```python
from build123d import *

# Parameters (mm, degrees)
SKETCH1_R           = 19.05
BOSS_EXTRUDE1_DEPTH = 12.7
SKETCH2_W           = 12.7
SKETCH2_H           = 2.54
SKETCH3_R           = 2.667
CUT_EXTRUDE1_DEPTH  = 30.784140075
BOSS_EXTRUDE2_DEPTH = 2.54
BOSS_EXTRUDE2_TAPER = 20
CIRPATTERN1_COUNT   = 6


with BuildPart() as part:
    # Sketch1 → Boss-Extrude1 (new body)
    with BuildSketch(Plane.XY):
        Circle(SKETCH1_R)
    extrude(amount=BOSS_EXTRUDE1_DEPTH)

    # Sketch2 → Cut-Revolve1 (revolve, cut)
    with BuildSketch(Plane(origin=(0, 0, 0), x_dir=(1, 0, 0), z_dir=(0, 1, 0)), mode=Mode.PRIVATE) as cut_revolve1_sk:
        with Locations((12.7, -6.35)):
            Rectangle(SKETCH2_W, SKETCH2_H)
    revolve(cut_revolve1_sk.sketch.rotate(Axis((0, 0, 0), (0, 0, 1)), 180), axis=Axis((0, 0, 0), (0, 0, 1)), mode=Mode.SUBTRACT)

    # Sketch3 → Cut-Extrude1 (cut, through all)
    with BuildSketch(Plane.XY.offset(12.7)):
        Circle(SKETCH3_R)
    extrude(amount=-CUT_EXTRUDE1_DEPTH, mode=Mode.SUBTRACT)

    # Sketch4 → Boss-Extrude2 (add)
    with BuildSketch(Plane(origin=(0, 0, 0), x_dir=(-1, 0, 0), z_dir=(0, 0, -1))):
        Polygon((-4.445, 3.050443212), (-2.54, 6.35), (-4.445, 9.649556788), (-8.255, 9.649556788), (-10.16, 6.35), (-8.255, 3.050443212), align=None)
    boss_extrude2 = extrude(amount=BOSS_EXTRUDE2_DEPTH, taper=BOSS_EXTRUDE2_TAPER)

    # CirPattern1: Boss-Extrude2 ×6 about axis
    cirpattern1_axis = Axis((0, 0, 0), (0, 0, 1))
    for i in range(1, CIRPATTERN1_COUNT):
        add(boss_extrude2.rotate(cirpattern1_axis, i * 360 / CIRPATTERN1_COUNT))


solid = part.part
```
Geometry: final body of the model. Coordinates: model frame, mm. A direction names the side the tool comes from. Give positions to 0.01 mm unless a question says otherwise; leave off trailing zeros. Order: outer loops, then holes, each group sorted by start corner. A loop starts at its lowest first (then second) coordinate and runs counter-clockwise, first axis right, second up. Notation, with made-up numbers: M 43.5,9.5 L 48.5,9.5 A18 ccw 48.5,31.5 Z; hole C -3.5,52 d8. An arc over 180 degrees is marked long. Answer as CSV lines item,"result". Start each with the question number.
1) Cut plane B-B (z = 1). Output: boundary loops of the cut face in (x, y), then the cut area to 3 significant figures.
2) First-contact query: P1, Ø4, axis at x = 8.5, z = 3.5, coming from the -Y side; P2, Ø6, axis at y = 6.5, z = 5, coming from the -X side; P3, Ø4, axis at x = 14, y = -11, coming from the -Z side. Flat tips, straight axial feed; report the tip coordinate or a pass-through.
3) Cut plane A-A (z = 6.25). Output: boundary loops of the cut face in (x, y).
4) Line query: line 1 (Z direction, x = 1.5, y = 7); line 2 (Y direction, x = 0, z = 5.25); line 3 (Y direction, x = 0, z = 8.5). Output: solid intervals per line, ascending. Write a range as from..to.
5) Set-up query: faces 1 (the flat face through (4, 0, 0)), 2 (the flat face through (-2, 9, -2.54)), 3 (the cylindrical face through (-2.93, 5.634, 6.332)). Return all of +Z, -Z, +X, -X, +Y, -Y with unobstructed straight access to the full face (end or side cutting, diameter ignored); none if empty.
6) Mould query, pull axis Z, two halves, no side actions, for faces 4 (the cylindrical face through (-15.12, -11.59, 2.5)), 5 (the flat face through (-5, -5, 7.62)), 6 (the flat face through (9, -2, -2.54)). Classes: +Z half, -Z half, draft (parallel to the pull), parting line (faces both ways), or undercut.
Findings below:
1,outline,"C 0,0 d38.1; hole C 0,0 d5.33"
1,area,"1,120 mm²"
2,P1,"stops at y = -17.91"
2,P2,"stops at x = -18.73"
2,P3,"stops at z = 0"
3,outline,"C 0,0 d12.7; hole C 0,0 d5.33"
4,line 1,"z = 0..5.08, 7.62..12.7"
4,line 2,"y = -6.35..-2.67, 2.67..6.35"
4,line 3,"y = -19.05..-2.67, 2.67..19.05"
5,face 1,"-Z"
5,face 2,"-Z, +X, -X, +Y, -Y"
5,face 3,"none"
6,face 4,"draft"
6,face 5,"undercut"
6,face 6,"-Z half"
